from build123d import *

# Parameters (mm, degrees)
F0_W          = 40
F0_H          = 20
F1_DEPTH      = 40
F3_START      = 2.5
F2_W          = 17.5
F2_H          = 15
F3_DEPTH      = 29.5
F4_W          = 20.5
F4_H          = 5.5
F4_W_2        = 7.25
F4_H_2        = 37.5
F5_DEPTH      = 25
F5_DEPTH_BACK = 25
F6_W          = 15
F6_H          = 6
F7_DEPTH      = 25
F7_DEPTH_BACK = 25
F8_R          = 2
F9_DEPTH      = 25
F9_DEPTH_BACK = 25
F10_SIZE      = 1.5
F12_R         = 3
F13_DEPTH     = 3


with BuildPart() as f1:
    # F0 (on Top) → F1 (new body)
    with BuildSketch(Plane.XY):
        Rectangle(F0_W, F0_H)
    extrude(amount=F1_DEPTH)

    # F2 (on Top) → F3 (cut)
    with BuildSketch(Plane.XY.offset(F3_START)):
        with Locations((-11.25, 0)):
            Rectangle(F2_W, F2_H)
        with Locations((11.25, 0)):
            Rectangle(F2_W, F2_H)
    extrude(amount=F3_DEPTH, mode=Mode.SUBTRACT)

    # F4 (on Front) → F5 (cut, two sides)
    with BuildSketch(Plane.XZ) as f5_sk:
        with Locations((0, 37.25)):
            Rectangle(F4_W, F4_H)
        with Locations((-16.375, 21.25)):
            Rectangle(F4_W_2, F4_H_2)
        with Locations((16.375, 21.25)):
            Rectangle(F4_W_2, F4_H_2)
    extrude(amount=-F5_DEPTH, mode=Mode.SUBTRACT)
    extrude(f5_sk.sketch, amount=F5_DEPTH_BACK, mode=Mode.SUBTRACT)

    # F6 (on Right) → F7 (cut, two sides)
    with BuildSketch(Plane.YZ) as f7_sk:
        with Locations((0, 29)):
            Rectangle(F6_W, F6_H)
    extrude(amount=-F7_DEPTH, mode=Mode.SUBTRACT)
    extrude(f7_sk.sketch, amount=F7_DEPTH_BACK, mode=Mode.SUBTRACT)

    # F8 (on Top) → F9 (cut, two sides)
    with BuildSketch(Plane.XY) as f9_sk:
        with Locations((-16, 0)):
            Circle(F8_R)
        with Locations((16, 0)):
            Circle(F8_R)
    extrude(amount=-F9_DEPTH, mode=Mode.SUBTRACT)
    extrude(f9_sk.sketch, amount=F9_DEPTH_BACK, mode=Mode.SUBTRACT)

    # F10
    f10_edges = [f1.edges().sort_by_distance(p)[0] for p in [
        (-18, 0, 2.5),
        (14, 0, 2.5),
    ]]
    chamfer(f10_edges, length=F10_SIZE)

    # F12 (on offset) → F13 (cut)
    with BuildSketch(Plane.XY.offset(34.5)):
        Circle(F12_R)
    extrude(amount=-F13_DEPTH, mode=Mode.SUBTRACT)


solid = f1.part
Geometry check sheet. Reference: the model listing, model coordinates, mm. A direction names the side the tool comes from. Give positions to 0.01 mm unless a question says otherwise; leave off trailing zeros. Loops run counter-clockwise (first coordinate to the right, second up) from the corner with the lowest first, then second, coordinate; pieces in that order, holes last. Notation, with made-up numbers: (57.25, 73) -> (67.25, 73) arc R36 cw to (67.25, 108) -> close; hole circle Ø7 at (-6, -30). An arc over 180 degrees is marked (long way). Answer in a Markdown table with one row per item. Add a question column.
1) Cross-section at B-B on x = -11.5. Record the boundary of the cut face in (y, z).
2) Draft check along Y on faces 1 (the face through (12.75, 0, 33)), 2 (the face through (0, 0, 26)). Enter one of: pulls with the +Y half, pulls with the -Y half, needs draft (parallel to the pull), parting line crosses it, or undercut.
3) Cross-section at D-D on x = -16. Record the boundary of the cut face in (y, z).
4) Cross-section at C-C on y = 4.5. Record the boundary of the cut face in (x, z), and give its area (3 significant figures).
5) Set-up check for faces 3 (the face through (-3, 0, 33)), 4 (the face through (-12.75, 0, 33)), 5 (the face through (10.25, 0, 37)), 6 (the face through (11, 0, 2.5)), 7 (the face through (-2.5, 0, 14)): record each of +Z, -Z, +X, -X, +Y, -Y from which the full face is reachable in a straight line by a thin tool's end or side.
6) Cross-section at A-A on y = 0. State how many separate pieces and enclosed holes the cut face has, and give its area (3 significant figures).
7) Gauge pin test, flat ends, axial feed: P1, Ø6, axis at y = -3.5, z = 28, coming from the +X side; P2, Ø3, axis at x = 16, y = 0, coming from the +Z side; P3, Ø1.6, axis at y = 3, z = 36.5, coming from the +X side; P4, Ø4.5, axis at y = -2, z = 13.5, coming from the -X side. Record the tip position at first contact, or that the pin passes through.
8) Material ranges on probe 1 along X at (y, z) = (0, 0.75); probe 2 along Y at (x, z) = (-9, 29); probe 3 along Z at (x, y) = (-3, 4), recorded low to high. Write a range as from..to.
Outcome:
| question | item | result |
|---|---|---|
| 1 | outline | (-10, 0) -> (10, 0) -> (10, 40) -> (-10, 40) -> close; hole (-7.5, 2.5) -> (7.5, 2.5) -> (7.5, 32) -> (-7.5, 32) -> close |
| 2 | face 1 | needs draft |
| 2 | face 2 | undercut |
| 3 | outline | (-10, 0) -> (-2, 0) -> (-2, 1) -> (-3.5, 2.5) -> (-10, 2.5) -> close; (2, 0) -> (10, 0) -> (10, 2.5) -> (3.5, 2.5) -> (2, 1) -> close |
| 4 | outline | (-20, 0) -> (20, 0) -> (20, 2.5) -> (2.5, 2.5) -> (2.5, 26) -> (-2.5, 26) -> (-2.5, 2.5) -> (-20, 2.5) -> close; (-12.75, 32) -> (12.75, 32) -> (12.75, 40) -> (10.25, 40) -> (10.25, 34.5) -> (-10.25, 34.5) -> (-10.25, 40) -> (-12.75, 40) -> close |
| 4 | area | 309 mm^2 |
| 5 | face 3 | +Z |
| 5 | face 4 | +Z, -X, +Y, -Y |
| 5 | face 5 | +Z, +Y, -Y |
| 5 | face 6 | +X |
| 5 | face 7 | -X |
| 6 | separate pieces | 5 |
| 6 | enclosed holes | 0 |
| 6 | area | 269 mm^2 |
| 7 | P1 | stops at x = 2.5 |
| 7 | P2 | passes through |
| 7 | P3 | stops at x = 12.75 |
| 7 | P4 | stops at x = -2.5 |
| 8 | probe 1 | x = -20..-18, -14..14, 18..20 |
| 8 | probe 2 | y = -10..-7.5, 7.5..10 |
| 8 | probe 3 | z = 0..2.5, 32..34.5 |
